For this review, take the finished solid that the model builds, in its own axes (mm). Coordinates: 2 decimals unless noted, no trailing zeros. Loops run counter-clockwise (first coordinate to the right, second up) from the corner with the lowest first, then second, coordinate; pieces in that order, holes last. Notation, with made-up numbers: (14.25, 76.25) - (36.25, 76.25) arc R14 cw to (36.25, 99.25) - close; hole circle Ø2 at (67, 67). An arc over 180 degrees is marked (long way). Answer as a JSON object with one key per item and string values. Group by question number.
Item 1: We need section B-B (z = 0). Give the boundary of the cut face in (x, y).
Item 2: Mouldability with a two-part tool opening along Z and no side actions: class faces 1 (the flat face through (0, 2, 10)), 2 (the flat face through (0, 5, 3)), 3 (the flat face through (0, 0, -5)), 4 (the cylindrical face through (-6.834, 7.465, -1.517)) as released by +Z, released by -Z, zero draft, split by the parting line, or undercut.
Item 3: Clearance check with flat-ended pins moving along their axes: pin 1 (1.5 mm diameter, centred on x = 14, z = -5.5, fed in from +Y); pin 2 (4 mm diameter, centred on y = 6, z = -1.5, fed in from -X); pin 3 (6 mm diameter, centred on y = 9, z = 7.5, fed in from +X); pin 4 (5 mm diameter, centred on y = 9, z = 3.5, fed in from +X). State where each tip first meets the part, or that it passes through.
Item 4: To check wall thickness, follow line 1 (X direction, y = 1.6, z = 0); line 2 (Z direction, x = -3, y = 0.5); line 3 (X direction, y = 7.75, z = 0). State the ranges of each line that lie inside material, in increasing order.
Item 5: We need section C-C (y = 3.25). Give the boundary of the cut face in (x, z), then the cut area to 3 significant figures.
Item 6: We need section A-A (x = -14). Give the boundary of the cut face in (y, z), then the cut area to 3 significant figures.
Item 7: We need section D-D (x = 0). Give the boundary of the cut face in (y, z).
from build123d import *

# Parameters (mm, degrees)
SKETCH1_W           = 40
SKETCH1_H           = 20
SKETCH1_R           = 1.5
BOSS_EXTRUDE1_DEPTH = 5
SKETCH2_R           = 7
BOSS_EXTRUDE2_DEPTH = 5


with BuildPart() as part:
    # Sketch1 → Boss-Extrude1 (new body)
    with BuildSketch(Plane(origin=(0, 0, 0), x_dir=(1, 0, 0), z_dir=(0, 1, 0))):
        Rectangle(SKETCH1_W, SKETCH1_H)
        with Locations(Location((14, 0, 0), (0, 0, 270))):
            Circle(SKETCH1_R, mode=Mode.SUBTRACT)
        with Locations(Location((-14, 0, 0), (0, 0, 270))):
            Circle(SKETCH1_R, mode=Mode.SUBTRACT)
        with BuildLine():
            Line((-2.645751311, -3), (2.645751311, -3))
            ThreePointArc((2.645751311, -3), (0, 4), (-2.645751311, -3))
        make_face(mode=Mode.SUBTRACT)
    extrude(amount=BOSS_EXTRUDE1_DEPTH)

    # Sketch2 → Boss-Extrude2 (add)
    with BuildSketch(Plane(origin=(0, 5, 0), x_dir=(1, 0, 0), z_dir=(0, 1, 0))):
        with Locations(Location((0, 0, 0), (0, 0, 270))):
            Circle(SKETCH2_R)
        with BuildLine():
            ThreePointArc((-2.645751311, -3), (0, 4), (2.645751311, -3))
            Line((2.645751311, -3), (-2.645751311, -3))
        make_face(mode=Mode.SUBTRACT)
    extrude(amount=BOSS_EXTRUDE2_DEPTH)


solid = part.part
Check sheet entries:
{
 "1": {"outline": "(-20, 0) - (-15.5, 0) - (-15.5, 5) - (-20, 5) - close; (-12.5, 0) - (-4, 0) - (-4, 10) - (-7, 10) - (-7, 5) - (-12.5, 5) - close; (4, 0) - (12.5, 0) - (12.5, 5) - (7, 5) - (7, 10) - (4, 10) - close; (15.5, 0) - (20, 0) - (20, 5) - (15.5, 5) - close"},
 "2": {"face 1": "released by +Z", "face 2": "undercut", "face 3": "zero draft", "face 4": "split by the parting line"},
 "3": {"pin 1": "stops at y = 5", "pin 2": "stops at x = -20", "pin 3": "stops at x = 5.36", "pin 4": "stops at x = 6.93"},
 "4": {"line 1": "x = -20 to -15.5, -12.5 to -4, 4 to 12.5, 15.5 to 20", "line 2": "z = -10 to -2.65, 2.65 to 10", "line 3": "x = -7 to -4, 4 to 7"},
 "5": {"outline": "(-20, -10) - (20, -10) - (20, 10) - (-20, 10) - close; hole circle Ø3 at (-14, 0); hole (-2.65, 3) arc R4 ccw (long way) to (2.65, 3) - close; hole circle Ø3 at (14, 0)", "area": "739 mm2"},
 "6": {"outline": "(0, -10) - (5, -10) - (5, -1.5) - (0, -1.5) - close; (0, 1.5) - (5, 1.5) - (5, 10) - (0, 10) - close", "area": "85.0 mm2"},
 "7": {"outline": "(0, -10) - (5, -10) - (5, -7) - (10, -7) - (10, -4) - (0, -4) - close; (0, 3) - (10, 3) - (10, 7) - (5, 7) - (5, 10) - (0, 10) - close"}
}
